Build history of the part. All positions in model axes, mm. A direction names the side the tool comes from. Coordinates: 2 decimals unless noted, no trailing zeros. Loops run counter-clockwise (first coordinate to the right, second up) from the corner with the lowest first, then second, coordinate; pieces in that order, holes last.
(1) Wall check: L1, parallel to Y at x = -29.5, z = 8.5; L2, parallel to Y at x = 0, z = 16; L3, parallel to Y at x = 59, z = 17. Give the ranges that are in metal, low to high.
(2) Tool access for faces 5 (the face through (13.09, 70.73, 12.52)), 6 (the face through (-28.08, 42.1, 12.52)), 7 (the face through (-68.01, 66.76, 12.52)), 8 (the face through (-44.868, -70.014, 12.522)): list every direction of +Z, -Z, +X, -X, +Y, -Y with a clear straight run to the whole face (end or side of a thin tool).
(3) Two-plate mould, pull along X, no slides. Class faces 1 (the face through (70.8, 51.51, 12.52)), 2 (the face through (-47.35, 56.76, 12.52)), 3 (the face through (0.4, 71.95, 12.52)), 4 (the face through (-71.748, -47.253, 12.522)): pulls with the +X half, pulls with the -X half, needs draft (parallel to the pull), parting line crosses it, or undercut.
(4) Flat gauge pins, fed straight in: P1, Ø16.5, axis at x = -55.79, y = 0, coming from the +Z side; P2, Ø10, axis at x = 54.5, z = 5, coming from the +Y side; P3, Ø1, axis at y = 17, z = 18, coming from the -X side; P4, Ø3, axis at x = -23, z = 13, coming from the +Y side. Where does each tip first touch, or does it go through?
(5) Slice it at A-A (x = 0). Give the cut face in (y, z).
(6) Slice it at B-B (z = 5.75). Give the number of separate pieces and of enclosed holes in the cut face, and give its area (3 significant figures).
from build123d import *

# Parameters (mm, degrees)
F0_R     = 10.7
F0_R_2   = 10.9
F0_R_3   = 9.1
F0_R_4   = 10.1
F0_R_5   = 9.3
F0_R_6   = 9.5
F0_R_7   = 11.1
F0_R_8   = 10.3
F0_R_9   = 9.7
F0_R_10  = 10.5
F0_R_11  = 9.9
F0_R_12  = 8
F0_R_13  = 8.225
F0_R_14  = 8.45
F0_R_15  = 7
F0_R_16  = 7.2
F0_R_17  = 7.4
F0_R_18  = 8.65
F0_R_19  = 8.85
F0_R_20  = 7.6
F0_R_21  = 7.8
F1_DEPTH = 25.4


with BuildPart() as f1:
    # F0 (on Top) → F1 (new body)
    with BuildSketch(Plane.XY):
        Polygon((-43.370046, 66.694871), (-71.039788, 73.835447), (-64.892714, 59.478019), (-74.194374, 47.642876), (-64.169625, 39.764069), (-74.194374, 33.27913), (-68.989453, 18.404532), (-75.21798, 12.435964), (-70.866387, 0), (-72.780757, -10.756556), (-65.846058, -21.280914), (-72.780757, -31.444447), (-68.989453, -42.279216), (-74.58584, -52.368706), (-68.060883, -60.507296), (-71.679206, -72.174512), (-59.155129, -67.792086), (-51.042687, -72.174512), (-38.51861, -67.792086), (-27.663881, -72.174512), (-19.667598, -52.368706), (-11.918255, -72.174512), (2.882631, -68.700455), (13.051437, -72.174512), (26.823167, -67.355507), (30.359259, -72.174512), (41.413072, -72.174512), (50.571952, -72.174512), (55.309299, -63.963108), (69.252096, -52.368706), (64.468175, -38.697239), (74.15197, -27.434214), (69.252096, -13.431376), (74.15197, -5.508246), (69.252096, 8.494591), (74.15197, 14.925677), (68.20149, 22.661304), (76.080737, 39.954469), (67.903966, 48.843425), (73.777615, 54.246476), (70.879206, 62.529534), (74.291575, 73.733234), (62.548533, 72.631314), (44.964856, 75.661271), (30.713456, 68.777539), (18.519877, 72.631314), (7.506575, 68.777539), (-6.904133, 75.213181), (-21.353263, 66.397347), (-28.986626, 72.697847), align=None)
        with Locations((-53.107839, -51.450886)):
            Circle(F0_R, mode=Mode.SUBTRACT)
        with Locations((0, -53.693082)):
            Circle(F0_R_2, mode=Mode.SUBTRACT)
        with Locations((-55.786539, 0)):
            Circle(F0_R_3, mode=Mode.SUBTRACT)
        with Locations((-36.131218, -25.825793)):
            Circle(F0_R_4, mode=Mode.SUBTRACT)
        with Locations((-28.625328, 0)):
            Circle(F0_R_5, mode=Mode.SUBTRACT)
        with Locations((0, -4.993503)):
            Circle(F0_R_6, mode=Mode.SUBTRACT)
        with Locations((36.900301, -55.614963)):
            Circle(F0_R_7, mode=Mode.SUBTRACT)
        with Locations((4.228305, -27.107049)):
            Circle(F0_R_8, mode=Mode.SUBTRACT)
        with Locations((27.933899, -6.271678)):
            Circle(F0_R_9, mode=Mode.SUBTRACT)
        with Locations((52.915979, -27.427362)):
            Circle(F0_R_10, mode=Mode.SUBTRACT)
        with Locations((58.059551, 0)):
            Circle(F0_R_11, mode=Mode.SUBTRACT)
        with Locations((-55.670351, 25.744705)):
            Circle(F0_R_12, mode=Mode.SUBTRACT)
        with Locations((-25.799653, 26.459009)):
            Circle(F0_R_13, mode=Mode.SUBTRACT)
        with Locations((0, 25.545178)):
            Circle(F0_R_14, mode=Mode.SUBTRACT)
        with Locations((-54.028157, 54.661482)):
            Circle(F0_R_15, mode=Mode.SUBTRACT)
        with Locations((-26.521808, 49.127601)):
            Circle(F0_R_16, mode=Mode.SUBTRACT)
        with Locations((0, 52.651051)):
            Circle(F0_R_17, mode=Mode.SUBTRACT)
        with Locations((27.931513, 25.104078)):
            Circle(F0_R_18, mode=Mode.SUBTRACT)
        with Locations((57.400368, 29.588468)):
            Circle(F0_R_19, mode=Mode.SUBTRACT)
        with Locations((27.6112, 49.447916)):
            Circle(F0_R_20, mode=Mode.SUBTRACT)
        with Locations((52.275352, 60.018267)):
            Circle(F0_R_21, mode=Mode.SUBTRACT)
    extrude(amount=F1_DEPTH)


solid = f1.part
Response values:
1. L1: y = -71.43 to -33.44, -18.21 to -9.26, 9.26 to 19.11, 33.8 to 42.57, 55.68 to 72.48
1. L2: y = -69.38 to -64.59, -42.79 to -36.5, -17.71 to -14.49, 4.51 to 17.1, 34 to 45.25, 60.05 to 72.13
1. L3: y = -60.89 to -35.99, -18.87 to -9.86, 9.86 to 20.88, 38.29 to 56.07, 63.97 to 73.24
2. face 5: +Z, -Z, +Y
2. face 6: +Z, -Z
2. face 7: +Z, -Z, -X
2. face 8: +Z, -Z, -Y
3. face 1: pulls with the +X half
3. face 2: undercut
3. face 3: undercut
3. face 4: pulls with the -X half
4. P1: passes through
4. P2: stops at y = 74.88
4. P3: stops at x = -70.98
4. P4: stops at y = 68.99
5. outline: (-69.38, 0) - (-64.59, 0) - (-64.59, 25.4) - (-69.38, 25.4) - close; (-42.79, 0) - (-36.5, 0) - (-36.5, 25.4) - (-42.79, 25.4) - close; (-17.71, 0) - (-14.49, 0) - (-14.49, 25.4) - (-17.71, 25.4) - close; (4.51, 0) - (17.1, 0) - (17.1, 25.4) - (4.51, 25.4) - close; (34, 0) - (45.25, 0) - (45.25, 25.4) - (34, 25.4) - close; (60.05, 0) - (72.13, 0) - (72.13, 25.4) - (60.05, 25.4) - close
6. separate pieces: 1
6. enclosed holes: 21
6. area: 14,200 mm2
